```python
from build123d import *

# Parameters (mm, degrees)
BOSS_EXTRUDE1_DEPTH      = 35
BOSS_EXTRUDE1_DEPTH_BACK = 35
SKETCH2_W                = 36
SKETCH2_H                = 20
HOLE1_D                  = 6.647
HOLE1_DEPTH              = 19.414509714
HOLE1_CSINK_D            = 8
HOLE1_CSINK_ANGLE        = 90
HOLE1_TIP                = 1.91882362
HOLE2_D                  = 6.647
HOLE2_DEPTH              = 19.414509714
HOLE2_CSINK_D            = 8
HOLE2_CSINK_ANGLE        = 90
HOLE2_TIP                = 1.91882362
HOLE3_D                  = 6.647
HOLE3_DEPTH              = 19.414509714
HOLE3_CSINK_D            = 8
HOLE3_CSINK_ANGLE        = 90
HOLE3_TIP                = 1.91882362
SKETCH26_R               = 10
CUT_EXTRUDE1_DEPTH       = 150
SKETCH27_R               = 10
CUT_EXTRUDE2_DEPTH       = 150
SKETCH28_W               = 177
SKETCH28_H               = 190
CUT_EXTRUDE3_DEPTH       = 70
CUT_EXTRUDE3_DEPTH_BACK  = 70
SKETCH29_R               = 4.5
CUT_EXTRUDE4_DEPTH       = 17.5


with BuildPart() as part:
    # Sketch1 → Boss-Extrude1 (new body, two sides)
    with BuildSketch(Plane(origin=(0, 0, 0), x_dir=(1, 0, 0), z_dir=(0, 1, 0))) as boss_extrude1_sk:
        with BuildLine():
            Line((-68.5, -71), (-35.25, -71))
            Line((-35.25, -71), (-35.25, -34))
            Line((-35.25, -34), (35.25, -34))
            Line((35.25, -34), (35.25, -71))
            Line((35.25, -71), (68.5, -71))
            Line((68.5, -71), (68.5, 79))
            Line((68.5, 79), (35.25, 79))
            Line((35.25, 79), (35.25, 0))
            ThreePointArc((35.25, 0), (34, -1.25), (32.75, 0))
            Line((32.75, 0), (-32.75, 0))
            ThreePointArc((-32.75, 0), (-34, -1.25), (-35.25, 0))
            Line((-35.25, 0), (-35.25, 79))
            Line((-35.25, 79), (-68.5, 79))
            Line((-68.5, 79), (-68.5, -71))
        make_face()
    extrude(amount=BOSS_EXTRUDE1_DEPTH)
    extrude(boss_extrude1_sk.sketch, amount=-BOSS_EXTRUDE1_DEPTH_BACK)

    # Sketch2 → Cut-Revolve1 (revolve, cut)
    with BuildSketch(Plane(origin=(0, 0, 0), x_dir=(0, 0, -1), z_dir=(1, 0, 0))):
        with Locations((-17, 10)):
            Rectangle(SKETCH2_W, SKETCH2_H)
    revolve(axis=Axis((0, 0, -1), (0, 0, 1)), mode=Mode.SUBTRACT)

    # Sketch3 → Cut-Revolve2 (revolve, cut)
    with BuildSketch(Plane(origin=(-23.25, 0, 0), x_dir=(0, 0, -1), z_dir=(1, 0, 0))):
        Polygon((-34, 23.25), (-34, 30.75), (-26, 30.75), (-26, 27.75), (0, 27.75), (0, 23.25), align=None)
    revolve(axis=Axis((-23.25, 23.25, 0), (0, 0, 1)), mode=Mode.SUBTRACT)

    # Sketch4 → Cut-Revolve3 (revolve, cut)
    with BuildSketch(Plane(origin=(-23.25, 0, 0), x_dir=(0, 0, -1), z_dir=(1, 0, 0))):
        Polygon((-34, -23.25), (-34, -15.75), (-26, -15.75), (-26, -18.75), (0, -18.75), (0, -23.25), align=None)
    revolve(axis=Axis((-23.25, -23.25, 0), (0, 0, 1)), mode=Mode.SUBTRACT)

    # Sketch5 → Cut-Revolve4 (revolve, cut)
    with BuildSketch(Plane(origin=(23.25, 0, 0), x_dir=(0, 0, -1), z_dir=(1, 0, 0))):
        Polygon((-34, 23.25), (-34, 30.75), (-26, 30.75), (-26, 27.75), (0, 27.75), (0, 23.25), align=None)
    revolve(axis=Axis((23.25, 23.25, 0), (0, 0, 1)), mode=Mode.SUBTRACT)

    # Sketch6 → Cut-Revolve5 (revolve, cut)
    with BuildSketch(Plane(origin=(23.25, 0, 0), x_dir=(0, 0, -1), z_dir=(1, 0, 0))):
        Polygon((-34, -23.25), (-34, -15.75), (-26, -15.75), (-26, -18.75), (0, -18.75), (0, -23.25), align=None)
    revolve(axis=Axis((23.25, -23.25, 0), (0, 0, 1)), mode=Mode.SUBTRACT)

    # Hole1
    with Locations(Plane(origin=(0, 35, 0), x_dir=(1, 0, 0), z_dir=(0, 1, 0))):
        with Locations((42.5, -18.8)):
            CounterSinkHole(HOLE1_D / 2, HOLE1_CSINK_D / 2, depth=HOLE1_DEPTH, counter_sink_angle=HOLE1_CSINK_ANGLE)
            with Locations((0, 0, -(HOLE1_DEPTH + HOLE1_TIP / 2))):  # 120° drill point
                Cone(0, HOLE1_D / 2, HOLE1_TIP, mode=Mode.SUBTRACT)

    # Hole2
    with Locations(Plane(origin=(0, 35, 0), x_dir=(1, 0, 0), z_dir=(0, 1, 0))):
        with Locations((-42.5, -18.8)):
            CounterSinkHole(HOLE2_D / 2, HOLE2_CSINK_D / 2, depth=HOLE2_DEPTH, counter_sink_angle=HOLE2_CSINK_ANGLE)
            with Locations((0, 0, -(HOLE2_DEPTH + HOLE2_TIP / 2))):  # 120° drill point
                Cone(0, HOLE2_D / 2, HOLE2_TIP, mode=Mode.SUBTRACT)

    # Sketch11 → Cut-Revolve6 (revolve, cut)
    with BuildSketch(Plane.XY.offset(18.8)):
        Polygon((48.5, 23.25), (50.41882362, 26.5735), (67.8235, 26.5735), (68.5, 27.25), (68.5, 23.25), align=None)
    revolve(axis=Axis((68.5, 23.25, 18.8), (-1, 0, 0)), mode=Mode.SUBTRACT)

    # Sketch12 → Cut-Revolve7 (revolve, cut)
    with BuildSketch(Plane.XY.offset(18.8)):
        Polygon((48.5, -23.25), (50.41882362, -19.9265), (67.8235, -19.9265), (68.5, -19.25), (68.5, -23.25), align=None)
    revolve(axis=Axis((68.5, -23.25, 18.8), (-1, 0, 0)), mode=Mode.SUBTRACT)

    # Sketch13 → Cut-Revolve8 (revolve, cut)
    with BuildSketch(Plane.XY.offset(18.8)):
        Polygon((-68.5, 23.25), (-68.5, 27.25), (-67.8235, 26.5735), (-50.41882362, 26.5735), (-48.5, 23.25), align=None)
    revolve(axis=Axis((-48.5, 23.25, 18.8), (-1, 0, 0)), mode=Mode.SUBTRACT)

    # Sketch14 → Cut-Revolve9 (revolve, cut)
    with BuildSketch(Plane.XY.offset(18.8)):
        Polygon((-68.5, -23.25), (-68.5, -19.25), (-67.8235, -19.9265), (-50.41882362, -19.9265), (-48.5, -23.25), align=None)
    revolve(axis=Axis((-48.5, -23.25, 18.8), (-1, 0, 0)), mode=Mode.SUBTRACT)

    # Hole3
    with Locations(Plane(origin=(0, 35, 0), x_dir=(1, 0, 0), z_dir=(0, 1, 0))):
        with Locations((42.5, 27.7)):
            CounterSinkHole(HOLE3_D / 2, HOLE3_CSINK_D / 2, depth=HOLE3_DEPTH, counter_sink_angle=HOLE3_CSINK_ANGLE)
            with Locations((0, 0, -(HOLE3_DEPTH + HOLE3_TIP / 2))):  # 120° drill point
                Cone(0, HOLE3_D / 2, HOLE3_TIP, mode=Mode.SUBTRACT)

    # Sketch17 → Cut-Revolve10 (revolve, cut)
    with BuildSketch(Plane.XY.offset(-27.7)):
        Polygon((-42.5, 35), (-38.5, 35), (-39.1765, 34.3235), (-39.1765, 15.585490286), (-42.5, 13.666666667), align=None)
    revolve(axis=Axis((-42.5, 13.666666667, -27.7), (0, 1, 0)), mode=Mode.SUBTRACT)

    # Sketch18 → Cut-Revolve11 (revolve, cut)
    with BuildSketch(Plane.XY.offset(-27.7)):
        Polygon((48.5, 23.25), (50.41882362, 26.5735), (67.8235, 26.5735), (68.5, 27.25), (68.5, 23.25), align=None)
    revolve(axis=Axis((68.5, 23.25, -27.7), (-1, 0, 0)), mode=Mode.SUBTRACT)

    # Sketch19 → Cut-Revolve12 (revolve, cut)
    with BuildSketch(Plane.XY.offset(-27.7)):
        Polygon((48.5, -23.25), (50.41882362, -19.9265), (67.8235, -19.9265), (68.5, -19.25), (68.5, -23.25), align=None)
    revolve(axis=Axis((68.5, -23.25, -27.7), (-1, 0, 0)), mode=Mode.SUBTRACT)

    # Sketch20 → Cut-Revolve13 (revolve, cut)
    with BuildSketch(Plane.XY.offset(-27.7)):
        Polygon((-68.5, 23.25), (-68.5, 27.25), (-67.8235, 26.5735), (-50.41882362, 26.5735), (-48.5, 23.25), align=None)
    revolve(axis=Axis((-48.5, 23.25, -27.7), (-1, 0, 0)), mode=Mode.SUBTRACT)

    # Sketch21 → Cut-Revolve14 (revolve, cut)
    with BuildSketch(Plane.XY.offset(-27.7)):
        Polygon((-68.5, -23.25), (-68.5, -19.25), (-67.8235, -19.9265), (-50.41882362, -19.9265), (-48.5, -23.25), align=None)
    revolve(axis=Axis((-48.5, -23.25, -27.7), (-1, 0, 0)), mode=Mode.SUBTRACT)

    # Sketch22 → Cut-Revolve15 (revolve, cut)
    with BuildSketch(Plane.XY.offset(-63)):
        Polygon((-68.5, 23.25), (-68.5, 27.25), (-67.8235, 26.5735), (-50.41882362, 26.5735), (-48.5, 23.25), align=None)
    revolve(axis=Axis((-48.5, 23.25, -63), (-1, 0, 0)), mode=Mode.SUBTRACT)

    # Sketch23 → Cut-Revolve16 (revolve, cut)
    with BuildSketch(Plane.XY.offset(-63)):
        Polygon((-68.5, -23.25), (-68.5, -19.25), (-67.8235, -19.9265), (-50.41882362, -19.9265), (-48.5, -23.25), align=None)
    revolve(axis=Axis((-48.5, -23.25, -63), (-1, 0, 0)), mode=Mode.SUBTRACT)

    # Sketch24 → Cut-Revolve17 (revolve, cut)
    with BuildSketch(Plane.XY.offset(37)):
        Polygon((-68.5, 23.25), (-68.5, 27.25), (-67.8235, 26.5735), (-50.41882362, 26.5735), (-48.5, 23.25), align=None)
    revolve(axis=Axis((-48.5, 23.25, 37), (-1, 0, 0)), mode=Mode.SUBTRACT)

    # Sketch25 → Cut-Revolve18 (revolve, cut)
    with BuildSketch(Plane.XY.offset(37)):
        Polygon((-68.5, -23.25), (-68.5, -19.25), (-67.8235, -19.9265), (-50.41882362, -19.9265), (-48.5, -23.25), align=None)
    revolve(axis=Axis((-48.5, -23.25, 37), (-1, 0, 0)), mode=Mode.SUBTRACT)

    # Sketch26 → Cut-Extrude1 (cut)
    with BuildSketch(Plane.XY.offset(-79)):
        with Locations((52, 0)):
            Circle(SKETCH26_R)
    extrude(amount=CUT_EXTRUDE1_DEPTH, mode=Mode.SUBTRACT)

    # Sketch27 → Cut-Extrude2 (cut)
    with BuildSketch(Plane.XY.offset(-79)):
        with Locations((-52, 0)):
            Circle(SKETCH27_R)
    extrude(amount=CUT_EXTRUDE2_DEPTH, mode=Mode.SUBTRACT)

    # Sketch28 → Cut-Extrude3 (cut, two sides)
    with BuildSketch(Plane(origin=(0, 0, 0), x_dir=(1, 0, 0), z_dir=(0, 1, 0))) as cut_extrude3_sk:
        with Locations((0, 4)):
            Rectangle(SKETCH28_W, SKETCH28_H)
        Polygon((-68.5, 18), (-68.2, 18), (-68.2, -9), (-68.5, -9), (-68.5, -47), (-68.2, -47), (-68.2, -71), (68.2, -71), (68.2, -31), (68.5, -31), (68.5, -9), (68.2, -9), (68.2, 18), (68.5, 18), (68.5, 40), (68.2, 40), (68.2, 79), (-68.5, 79), (-68.5, 52), (-68.2, 52), (-68.2, 40), (-68.5, 40), align=None, mode=Mode.SUBTRACT)
    extrude(amount=CUT_EXTRUDE3_DEPTH, mode=Mode.SUBTRACT)
    extrude(cut_extrude3_sk.sketch, amount=-CUT_EXTRUDE3_DEPTH_BACK, mode=Mode.SUBTRACT)

    # Sketch29 → Cut-Extrude4 (cut)
    with BuildSketch(Plane(origin=(0, 35, 0), x_dir=(1, 0, 0), z_dir=(0, 1, 0))):
        with Locations((-42.5, 42.7)):
            Circle(SKETCH29_R)
        with Locations((42.5, -33.8)):
            Circle(SKETCH29_R)
    extrude(amount=-CUT_EXTRUDE4_DEPTH, mode=Mode.SUBTRACT)


solid = part.part
```
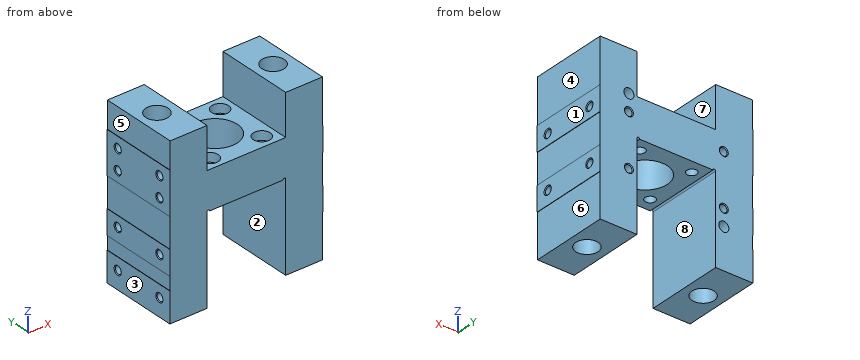
Work out the finished part from the listing and answer in its coordinate system (mm). Face numbers are marked on the shaded views. A direction names the side the tool comes from. Coordinates: 2 decimals unless noted, no trailing zeros. Loops run counter-clockwise (first coordinate to the right, second up) from the corner with the lowest first, then second, coordinate; pieces in that order, holes last.
1) For a pull along X with two mould halves and no side action, classify the marked faces 1, 2 and 3 as +X half, -X half, draft (parallel to the pull), parting line (faces both ways), or undercut.
Results:
face 1: +X half
face 2: undercut
face 3: -X half
2) Section C-C (x = 23.25) is taken. Give the vertices of the cut face in (y, z).
Results:
outline: (-35, 0) - (-27.75, 0) - (-27.75, 26) - (-30.75, 26) - (-30.75, 34) - (-35, 34) - close; (-18.75, 0) - (18.75, 0) - (18.75, 26) - (15.75, 26) - (15.75, 34) - (-15.75, 34) - (-15.75, 26) - (-18.75, 26) - close; (27.75, 0) - (35, 0) - (35, 34) - (30.75, 34) - (30.75, 26) - (27.75, 26) - close
3) Section B-B (x = 0) is taken. Give the vertices of the cut face in (y, z), plus the area to 3 significant figures.
Results:
outline: (-35, 0) - (-20, 0) - (-20, 34) - (-35, 34) - close; (20, 0) - (35, 0) - (35, 34) - (20, 34) - close
area: 1,020 mm2
4) For the marked faces 4, 5, 6, 7 and 8, determine the directions among +Z, -Z, +X, -X, +Y, -Y from which every point of the face is accessible in a straight line to the end or side of a thin tool.
Results:
face 4: +Z, +X, +Y, -Y
face 5: +Z, -X, +Y, -Y
face 6: -Z, +X, +Y, -Y
face 7: +Z, +Y, -Y
face 8: -Z, +Y, -Y
5) Flat-ended cylindrical pins translate along their axes: pin 1 (10 mm diameter, centred on x = -11, y = 24, fed in from -Z); pin 2 (1.5 mm diameter, centred on x = -25, y = 15, fed in from +Z); pin 3 (7.5 mm diameter, centred on x = -25, y = 22, fed in from +Z). Find the tip coordinate at first contact, or state that the pin passes through.
Results:
pin 1: stops at z = 0
pin 2: stops at z = 34
pin 3: stops at z = 26
6) Consider probe 1 along X at (y, z) = (24, 33.8); probe 2 along Y at (x, z) = (-23.25, 30.75); probe 3 along Z at (x, y) = (-42.5, 28.25). Determine where each line is inside the solid, lowest interval first.
Results:
probe 1: x = -50.4 to -30.71, -15.79 to 15.79, 30.71 to 38, 47 to 68.2
probe 2: y = -35 to -30.75, -15.75 to 15.75, 30.75 to 35
probe 3: z = -79 to -47.2, -38.2 to -31.02, -24.38 to 15.48, 22.12 to 71
7) Section A-A (z = -57) is taken. Give the vertices of the cut face in (x, y).
Results:
outline: (-68.5, -35) - (-35.25, -35) - (-35.25, 35) - (-68.5, 35) - close; (35.25, -35) - (68.2, -35) - (68.2, 35) - (35.25, 35) - close; hole circle Ø20 at (-52, 0); hole circle Ø20 at (52, 0)
